Can you work these out from the model? Positions are in its coordinate system, mm. Face numbers are marked on the shaded views. A direction names the side the tool comes from. Coordinates: 2 decimals unless noted, no trailing zeros. Order: outer loops, then holes, each group sorted by start corner. A loop starts at its lowest first (then second) coordinate and runs counter-clockwise, first axis right, second up.
```python
from build123d import *

# Parameters (mm, degrees)
SKETCH1_W           = 9
SKETCH1_H           = 10.8
BOSS_EXTRUDE1_DEPTH = 2.9
BOSS_EXTRUDE2_DEPTH = 10.9
SKETCH3_R           = 3.2
CUT_EXTRUDE1_DEPTH  = 9.54
SKETCH4_R           = 0.875
BOSS_EXTRUDE3_DEPTH = 7.87
FILLET1_R           = 0.4
SKETCH5_W           = 2.54
SKETCH5_H           = 0.25
SKETCH5_W_2         = 2.3
SKETCH5_H_2         = 0.35
SKETCH5_W_3         = 0.35
SKETCH5_H_3         = 2.2
BOSS_EXTRUDE4_DEPTH = 4.3
CUT_EXTRUDE2_START  = -0.25
SKETCH6_R           = 0.65
CUT_EXTRUDE2_DEPTH  = 0.25
SKETCH7_R           = 0.65
CUT_EXTRUDE3_DEPTH  = 18.881265336
CUT_EXTRUDE5_START  = -0.35
SKETCH9_R           = 0.65
CUT_EXTRUDE5_DEPTH  = 0.35


with BuildPart() as part:
    # Sketch1 → Boss-Extrude1 (new body)
    with BuildSketch(Plane.XY):
        with Locations((4.5, 5.4)):
            Rectangle(SKETCH1_W, SKETCH1_H)
    extrude(amount=BOSS_EXTRUDE1_DEPTH)

    # Sketch2 → Boss-Extrude2 (add)
    with BuildSketch(Plane(origin=(0, 0, 0), x_dir=(-1, 0, 0), z_dir=(0, 0, -1))):
        with BuildLine():
            Line((-9, 0), (0, 0))
            Line((0, 0), (0, 6.24))
            Line((0, 6.24), (-0.50005, 6.24))
            ThreePointArc((-0.50005, 6.24), (-4.5, 10.26), (-8.49995, 6.24))
            Line((-8.49995, 6.24), (-9, 6.24))
            Line((-9, 6.24), (-9, 0))
        make_face()
    extrude(amount=BOSS_EXTRUDE2_DEPTH)

    # Sketch3 → Cut-Extrude1 (cut)
    with BuildSketch(Plane.XY.offset(2.9)):
        with Locations((4.5, 6.26)):
            Circle(SKETCH3_R)
    extrude(amount=-CUT_EXTRUDE1_DEPTH, mode=Mode.SUBTRACT)

    # Sketch4 → Boss-Extrude3 (add)
    with BuildSketch(Plane.XY.offset(-6.64)):
        with Locations(Location((4.5, 6.26, 0), (0, 0, 180))):
            Circle(SKETCH4_R)
    extrude(amount=BOSS_EXTRUDE3_DEPTH)

    # Fillet1
    fillet1_edges = [part.edges().sort_by_distance(p)[0] for p in [
        (5.375, 6.26, 1.23),
    ]]
    fillet(fillet1_edges, radius=FILLET1_R)

    # Sketch5 → Boss-Extrude4 (add)
    with BuildSketch(Plane.XZ):
        with Locations((4.5, -4.425)):
            Rectangle(SKETCH5_W, SKETCH5_H)
        with Locations((4.5, -10.73)):
            Rectangle(SKETCH5_W_2, SKETCH5_H_2)
        with Locations((9, -7.955)):
            Rectangle(SKETCH5_W_3, SKETCH5_H_3)
    extrude(amount=BOSS_EXTRUDE4_DEPTH)

    # Sketch6 → Cut-Extrude2 (cut)
    with BuildSketch(Plane.XY.offset(-4.3).offset(CUT_EXTRUDE2_START)):
        with Locations((4.5, -3.03)):
            Circle(SKETCH6_R)
        with BuildLine():
            Line((3.23, -3.03), (2.98145415, -3.03))
            Line((2.98145415, -3.03), (2.98145415, -4.481636856))
            Line((2.98145415, -4.481636856), (5.931605951, -4.481636856))
            Line((5.931605951, -4.481636856), (5.931605951, -3.03))
            Line((5.931605951, -3.03), (5.77, -3.03))
            ThreePointArc((5.77, -3.03), (4.5, -4.3), (3.23, -3.03))
        make_face()
    extrude(amount=CUT_EXTRUDE2_DEPTH, mode=Mode.SUBTRACT)

    # Sketch7 → Cut-Extrude3 (cut, through all)
    with BuildSketch(Plane(origin=(9.175, 0, 0), x_dir=(0, 0, -1), z_dir=(1, 0, 0))):
        with Locations((7.955, -3.2)):
            Circle(SKETCH7_R)
        with BuildLine():
            Line((6.855, -3.2), (6.537099377, -3.2))
            Line((6.537099377, -3.2), (6.537099377, -4.556833282))
            Line((6.537099377, -4.556833282), (9.415825045, -4.556833282))
            Line((9.415825045, -4.556833282), (9.415825045, -3.2))
            Line((9.415825045, -3.2), (9.055, -3.2))
            ThreePointArc((9.055, -3.2), (7.955, -4.3), (6.855, -3.2))
        make_face()
    extrude(amount=-CUT_EXTRUDE3_DEPTH, mode=Mode.SUBTRACT)

    # Sketch9 → Cut-Extrude5 (cut)
    with BuildSketch(Plane(origin=(0, 0, -10.905), x_dir=(-1, 0, 0), z_dir=(0, 0, -1)).offset(CUT_EXTRUDE5_START)):
        with Locations((-4.5, -3.15)):
            Circle(SKETCH9_R)
        with BuildLine():
            Line((-5.65, -3.15), (-6.063372646, -3.15))
            Line((-6.063372646, -3.15), (-6.063372646, -4.563001678))
            Line((-6.063372646, -4.563001678), (-3.002045836, -4.563001678))
            Line((-3.002045836, -4.563001678), (-3.002045836, -3.15))
            Line((-3.002045836, -3.15), (-3.35, -3.15))
            ThreePointArc((-3.35, -3.15), (-4.5, -4.3), (-5.65, -3.15))
        make_face()
    extrude(amount=CUT_EXTRUDE5_DEPTH, mode=Mode.SUBTRACT)


solid = part.part
```
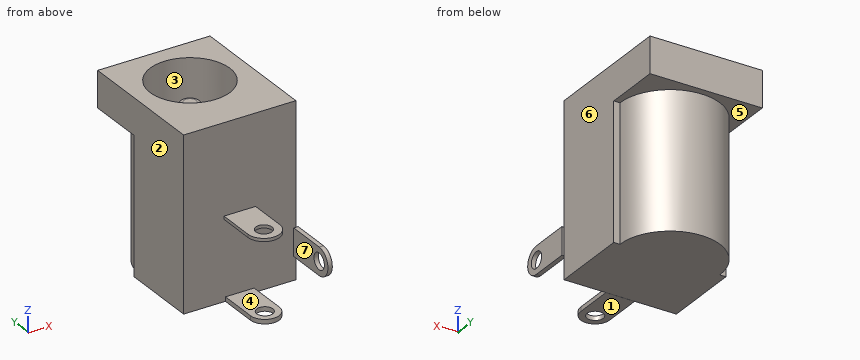
1. On a 3-axis mill with a long thin cutter (end or side, diameter ignored), from which of +Z, -Z, +X, -X, +Y, -Y can I reach the whole of each face in a straight line? I mean the marked faces 4, 5, 6 and 7. Say none if no direction works.
Completed:
face 4: +X, -X, -Y
face 5: -Z, +Y
face 6: +Z, -Z, +X, +Y
face 7: +Z, -Z, -X, -Y
2. Imagine slicing it at A-A on z = -1.25. Please give me the cut outline in (x, y) (3 decimals), then the cut area to 3 significant figures.
Completed:
outline: (0, 0) - (9, 0) - (9, 6.24) - (8.5, 6.24) arc R4 ccw (long way) to (0.5, 6.24) - (0, 6.24) - close; circle Ø1.75 at (4.5, 6.26); hole circle Ø6.4 at (4.5, 6.26)
area: 51.7 mm2
3. Imagine slicing it at D-D on x = 0.75. Please give me the cut outline in (y, z), then the cut area to 3 significant figures.
Completed:
outline: (0, -10.9) - (7.65, -10.9) - (7.65, 0) - (10.8, 0) - (10.8, 2.9) - (0, 2.9) - close
area: 115 mm2
4. Imagine slicing it at C-C on x = 7. Please give me the cut outline in (y, z), then the cut area to 3 significant figures.
Completed:
outline: (0, -10.9) - (9.38, -10.9) - (9.38, 0) - (10.8, 0) - (10.8, 2.9) - (8.26, 2.9) - (8.26, -6.64) - (4.26, -6.64) - (4.26, 2.9) - (0, 2.9) - close
area: 95.5 mm2
5. Imagine slicing it at B-B on x = 4.5. Give the number of separate pieces and of enclosed holes in the cut face, then the cut area to 3 significant figures.
Completed:
separate pieces: 3
enclosed holes: 0
area: 97.6 mm2
6. I'm going to push flat-ended pins straight in: pin 1 (4 mm diameter, centred on x = 1, z = -1, fed in from -Y); pin 2 (2 mm diameter, centred on x = 5, y = -2, fed in from +Z); pin 3 (3 mm diameter, centred on x = 4.5, z = -8, fed in from +Y); pin 4 (0.8 mm diameter, centred on x = 4.5, y = -3.15, fed in from +Z). Where does each tip first touch, or does it pass through?
Completed:
pin 1: stops at y = 0
pin 2: stops at z = -4.3
pin 3: stops at y = 10.26
pin 4: passes through
7. Thinking about a two-plate mould opening in X: for the marked faces 1, 2 and 3, which applies, pulls with the +X half, pulls with the -X half, needs draft (parallel to the pull), parting line crosses it, or undercut?
Completed:
face 1: needs draft
face 2: pulls with the -X half
face 3: undercut
8. Please list where these lines run through material, in increasing order: probe 1 along Y at (x, z) = (4.5, -2.75) (3 decimals); probe 2 along Y at (x, z) = (4.5, -4.35) (3 decimals); probe 3 along Y at (x, z) = (5, -2.5).
Completed:
probe 1: y = 0 to 3.06, 5.385 to 7.135, 9.46 to 10.26
probe 2: y = -4.3 to -3.68, -2.38 to 3.06, 5.385 to 7.135, 9.46 to 10.26
probe 3: y = 0 to 3.1, 5.54 to 6.98, 9.42 to 10.23
